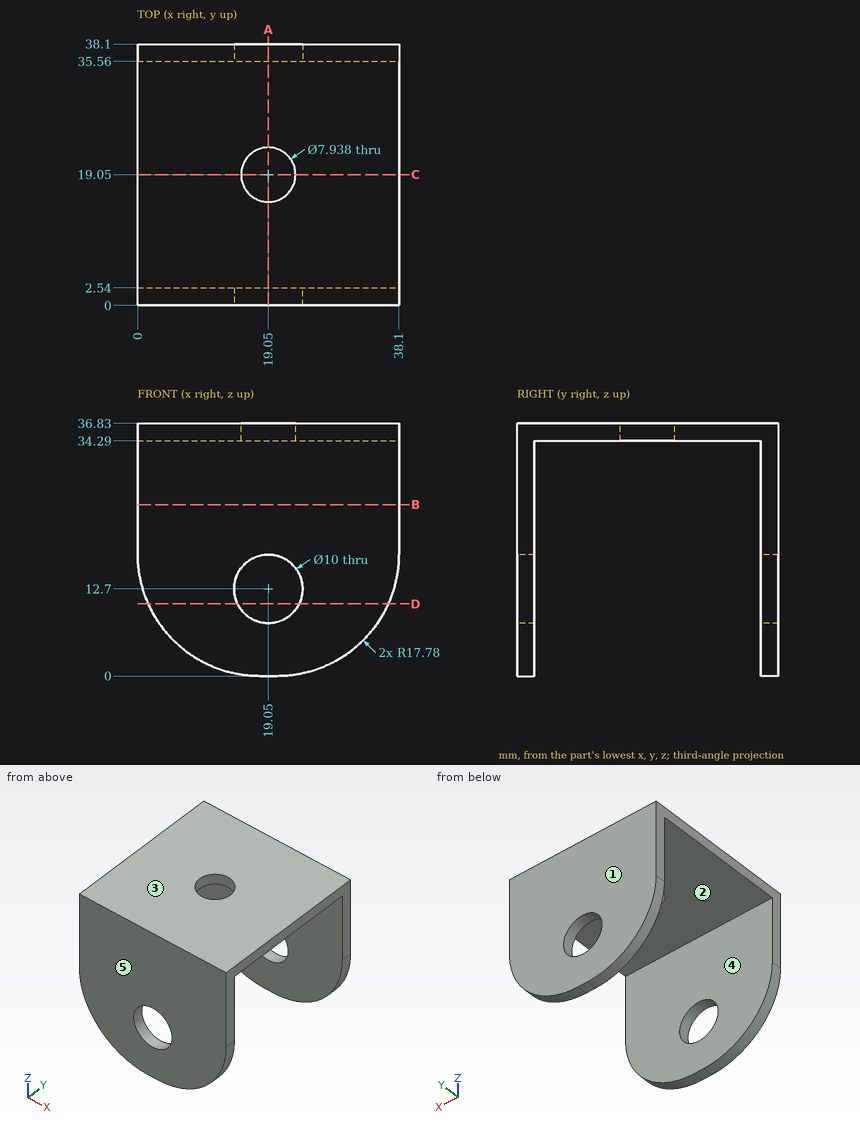
Geometry check sheet. Reference: drawing and pictorial views, mm from the part's lowest x, y, z. A direction names the side the tool comes from. Round coordinates to 2 decimals unless told otherwise and drop trailing zeros. Order: outer loops, then holes, each group sorted by start corner. A loop starts at its lowest first (then second) coordinate and runs counter-clockwise, first axis right, second up. Notation, with made-up numbers: M 89,10 L 104,10 A13 ccw 104,14 Z; hole C 13,74.25 d7. An arc over 180 degrees is marked long. Answer as CSV lines item,"result".
1) Gauge pin test, flat end, axial feed: pin 1 Ø9 at (x, y) = (19.05, 19.05) entering from -Z. Record the tip position at first contact, or that the pin passes through.
Entries:
pin 1,"z = 34.29"
2) Thickness scan on probe 1 along Y at (x, z) = (13.5, 24.5); probe 2 along Y at (x, z) = (19, 35); probe 3 along Z at (x, y) = (19, 37). Record the ranges inside material, lowest first. Write a range as [from, to].
Entries:
probe 1,"[0, 2.54], [35.56, 38.1]"
probe 2,"[0, 15.08], [23.02, 38.1]"
probe 3,"[0, 7.7], [17.7, 36.83]"
3) Sectioned sample at A-A on x = 19.05. Record the cut outline in (y, z), and give its area (3 significant figures).
Entries:
outline,"M 0,0 L 2.54,0 L 2.54,7.7 L 0,7.7 Z; M 0,17.7 L 2.54,17.7 L 2.54,34.29 L 15.08,34.29 L 15.08,36.83 L 0,36.83 Z; M 23.02,34.29 L 35.56,34.29 L 35.56,17.7 L 38.1,17.7 L 38.1,36.83 L 23.02,36.83 Z; M 35.56,0 L 38.1,0 L 38.1,7.7 L 35.56,7.7 Z"
area,"200 mm2"
4) Sectioned sample at B-B on z = 25. Record the cut outline in (x, y).
Entries:
outline,"M 0,0 L 38.1,0 L 38.1,2.54 L 0,2.54 Z; M 0,35.56 L 38.1,35.56 L 38.1,38.1 L 0,38.1 Z"
5) Tool access check on the marked faces 1 and 2. Record the directions out of +Z, -Z, +X, -X, +Y, -Y that give a thin tool (end or side, any length) a straight path to the whole face; none if there is none.
Entries:
face 1,"+Z, -Z, +X, -X, +Y"
face 2,"-Z, +X, -X"
6) Sectioned sample at D-D on z = 10.5. Record the cut outline in (x, y), and give its area (3 significant figures).
Entries:
outline,"M 1.56,0 L 14.56,0 L 14.56,2.54 L 1.56,2.54 Z; M 1.56,35.56 L 14.56,35.56 L 14.56,38.1 L 1.56,38.1 Z; M 23.54,0 L 36.54,0 L 36.54,2.54 L 23.54,2.54 Z; M 23.54,35.56 L 36.54,35.56 L 36.54,38.1 L 23.54,38.1 Z"
area,"132 mm2"
7) Sectioned sample at C-C on y = 19.05. Record the cut outline in (x, z).
Entries:
outline,"M 0,34.29 L 15.08,34.29 L 15.08,36.83 L 0,36.83 Z; M 23.02,34.29 L 38.1,34.29 L 38.1,36.83 L 23.02,36.83 Z"
8) Mould release check, pull along Y, two halves, no side actions. Record for the marked faces 3, 4 and 5: +Y half, -Y half, draft (parallel to the pull), parting line (faces both ways), or undercut.
Entries:
face 3,"draft"
face 4,"undercut"
face 5,"-Y half"
